Build history of the part. All positions in model axes, mm. Face numbers are marked on the shaded views. Round coordinates to 2 decimals unless told otherwise and drop trailing zeros. Write each loop counter-clockwise with the first axis right and the second up, starting at its lowest first coordinate (ties: lowest second). Pieces come first, ordered by that corner, then holes. Notation, with made-up numbers: (39, 68.5) -> (87, 68.5) arc R17 cw to (87, 88.5) -> close; hole circle Ø1 at (-14.75, 73). An arc over 180 degrees is marked (long way). Answer in a Markdown table with one row per item.
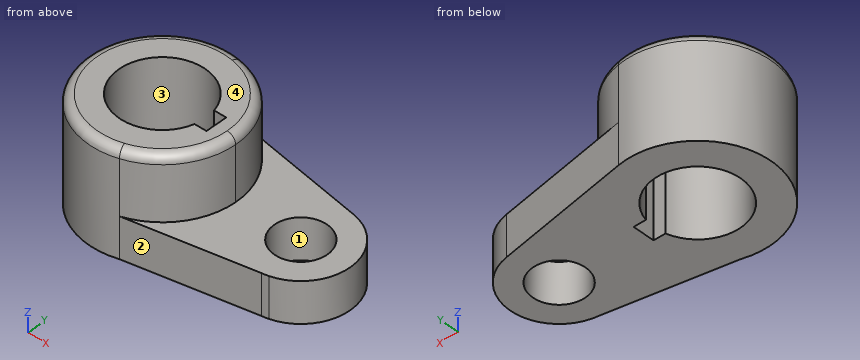
```python
from build123d import *

# Parameters (mm, degrees)
F0_R     = 16.762017
F0_R_2   = 10.2415
F1_DEPTH = 15.7734
F2_DEPTH = 40.2336
F4_DEPTH = 57.912
F5_R     = 3.302


with BuildPart() as f1:
    # F0 (on Top) → F1 (new body)
    with BuildSketch(Plane.XY):
        with BuildLine():
            ThreePointArc((8.398844, -27.312818), (22.98399, -16.978422), (28.575, 0))
            ThreePointArc((28.575, 0), (21.916025, 18.336262), (5.042647, 28.126541))
            ThreePointArc((5.042647, 28.126541), (-28.522782, -1.726717), (8.398844, -27.312818))
        make_face()
        Circle(F0_R, mode=Mode.SUBTRACT)
        with BuildLine():
            ThreePointArc((5.042647, 28.126541), (21.916025, 18.336262), (28.575, 0))
            ThreePointArc((28.575, 0), (22.98399, -16.978422), (8.398844, -27.312818))
            Line((8.398844, -27.312818), (55.972016, -18.945037))
            Line((55.972016, -18.945037), (58.562435, -18.489401))
            ThreePointArc((58.562435, -18.489401), (73.014691, 0.626641), (57.336765, 18.751028))
            Line((57.336765, 18.751028), (5.042647, 28.126541))
        make_face()
        with Locations((53.975, 0)):
            Circle(F0_R_2, mode=Mode.SUBTRACT)
        with BuildLine():
            Line((58.562435, -18.489401), (55.972016, -18.945037))
            ThreePointArc((55.972016, -18.945037), (57.275098, -18.761979), (58.562435, -18.489401))
        make_face()
    extrude(amount=F1_DEPTH)

    # F0 (on Top) → F2 (join)
    with BuildSketch(Plane.XY):
        with BuildLine():
            ThreePointArc((8.398844, -27.312818), (22.98399, -16.978422), (28.575, 0))
            ThreePointArc((28.575, 0), (21.916025, 18.336262), (5.042647, 28.126541))
            ThreePointArc((5.042647, 28.126541), (-28.522782, -1.726717), (8.398844, -27.312818))
        make_face()
        Circle(F0_R, mode=Mode.SUBTRACT)
    extrude(amount=F2_DEPTH)

    # F3 (on face) → F4 (cut)
    with BuildSketch(Plane.XY.offset(40.2336)):
        with BuildLine():
            Line((20.948661, 4.355739), (16.18619, 4.355739))
            ThreePointArc((16.18619, 4.355739), (16.617437, 2.196818), (16.762017, 0))
            ThreePointArc((16.762017, 0), (16.6366, -2.046642), (16.262227, -4.062657))
            Line((16.262227, -4.062657), (20.948661, -4.062657))
            Line((20.948661, -4.062657), (20.948661, 4.355739))
        make_face()
    extrude(amount=-F4_DEPTH, mode=Mode.SUBTRACT)

    # F5
    f5_edges = [f1.edges().sort_by_distance(p)[0] for p in [
        (-8.398844, 27.312818, 40.2336),
    ]]
    fillet(f5_edges, radius=F5_R)


solid = f1.part
```
Q1. Saw through at B-B on z = 13. State how many separate pieces and enclosed holes the cut face has, plus the area to 3 significant figures.
A:
| item | result |
|---|---|
| separate pieces | 1 |
| enclosed holes | 2 |
| area | 3,210 mm² |
Q2. Two-plate mould, pull along X, no slides. Class the marked faces 1, 2, 3 and 4: released by +X, released by -X, zero draft, split by the parting line, or undercut.
A:
| item | result |
|---|---|
| face 1 | undercut |
| face 2 | released by +X |
| face 3 | undercut |
| face 4 | zero draft |
Q3. Drop flat-ended pins along their axis: P1, Ø8, axis at x = 61.5, y = 15, coming from the +Z side; P2, Ø1.4, axis at x = 19, z = 17, coming from the +Y side; P3, Ø6, axis at y = 2, z = 13.5, coming from the -X side (3 decimals). Give the stop position or say it passes through.
A:
| item | result |
|---|---|
| P1 | z = 15.77 |
| P2 | y = 21.95 |
| P3 | x = -28.575 |
Q4. Wall check: line 1 (X direction, y = 7.5, z = 14.5); line 2 (X direction, y = 0, z = 21) (3 decimals); line 3 (Y direction, x = 0, z = 15.5) (3 decimals). Give the ranges that are in metal, low to high. Write a range as [from, to].
A:
| item | result |
|---|---|
| line 1 | [-27.57, -14.99], [14.99, 47], [60.95, 71.49] |
| line 2 | [-28.575, -16.762], [20.949, 28.575] |
| line 3 | [-28.575, -16.762], [16.762, 28.575] |
Q5. Saw through at A-A on z = 24.5. Write the cut outline in (x, y) (3 decimals).
A:
| item | result |
|---|---|
| outline | (5.043, 28.127) arc R28.575 ccw (long way) to (28.575, 0) arc R28.575 ccw to start; hole (16.186, 4.356) arc R16.762 ccw (long way) to (16.262, -4.063) -> (20.949, -4.063) -> (20.949, 4.356) -> close |
